Check sheet for the drawn part. Datum: minimum x, y, z corner. Units: mm. Coordinates: 2 decimals unless noted, no trailing zeros. Order: outer loops, then holes, each group sorted by start corner. A loop starts at its lowest first (then second) coordinate and runs counter-clockwise, first axis right, second up. Notation, with made-up numbers: (67, 52.5) - (76, 52.5) arc R17 ccw to (76, 68.5) - close; hole circle Ø11 at (-7.5, -40). An arc over 180 degrees is marked (long way). Put each result on its own line as item: value.
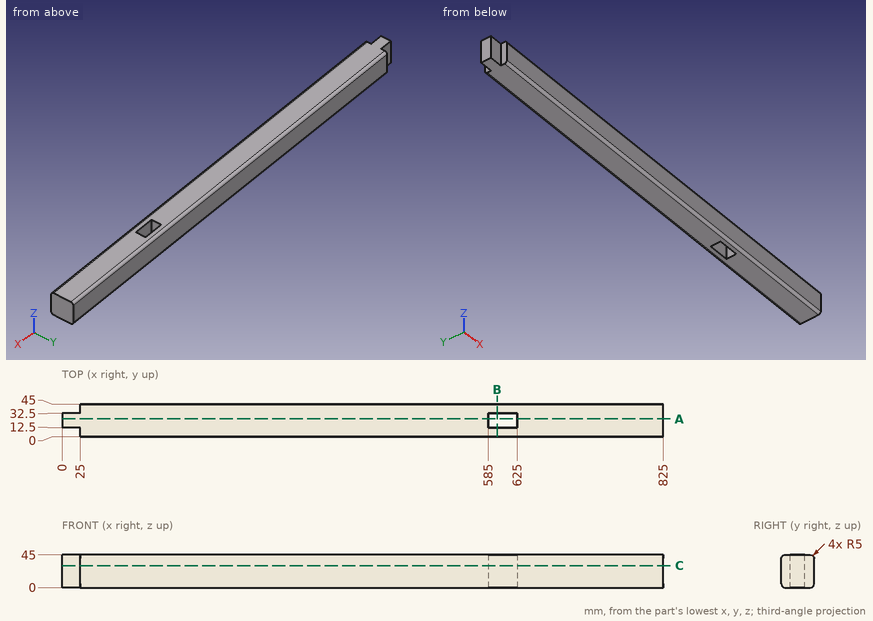
Q1. Depth check by flat-ended pin: pin 1 Ø2 at (y, z) = (32, 6) entering from -X; pin 2 Ø6 at (y, z) = (38.5, 25) entering from -X; pin 3 Ø12.5 at (x, z) = (15.5, 30) entering from -Y. Enter the tip coordinate at first touch or a pass-through.
Answer block:
pin 1: stops at x = 0
pin 2: stops at x = 25
pin 3: stops at y = 12.5
Q2. Section check B-B on x = 597. Record the boundary of the cut face in (y, z), then the cut area to 3 significant figures.
Answer block:
outline: (0, 5) arc R5 ccw to (5, 0) - (12.5, 0) - (12.5, 45) - (5, 45) arc R5 ccw to (0, 40) - close; (32.5, 0) - (40, 0) arc R5 ccw to (45, 5) - (45, 40) arc R5 ccw to (40, 45) - (32.5, 45) - close
area: 1,100 mm^2
Q3. Section check C-C on z = 30. Record the boundary of the cut face in (x, y).
Answer block:
outline: (0, 12.5) - (25, 12.5) - (25, 0) - (825, 0) - (825, 45) - (25, 45) - (25, 32.5) - (0, 32.5) - close; hole (585, 12.5) - (625, 12.5) - (625, 32.5) - (585, 32.5) - close
Q4. Thickness scan on L1, parallel to X at y = 23.5, z = 10; L2, parallel to X at y = 6, z = 37.5; L3, parallel to Y at x = 448, z = 41. Record the ranges inside material, lowest first. Write a range as [from, to].
Answer block:
L1: x = [0, 585], [625, 825]
L2: x = [25, 825]
L3: y = [0.1, 44.9]
Q5. Section check A-A on y = 24.5. Record the boundary of the cut face in (x, z), then the cut area to 3 significant figures.
Answer block:
outline: (0, 0) - (585, 0) - (585, 45) - (0, 45) - close; (625, 0) - (825, 0) - (825, 45) - (625, 45) - close
area: 35,300 mm^2
